Input: part model. Units: mm. Frame: model coordinates. Round coordinates to 2 decimals unless told otherwise and drop trailing zeros. Loops run counter-clockwise (first coordinate to the right, second up) from the corner with the lowest first, then second, coordinate; pieces in that order, holes last.
(1) Cut plane B-B, the plane x = 50.8. Output: boundary loops of the cut face in (y, z).
(2) Line query: line 1 (X direction, y = 22, z = 25.4); line 2 (X direction, y = 34.5, z = -27.5); line 3 (Z direction, x = -49, y = 22.5). Output: solid intervals per line, ascending.
(3) Cut plane A-A, the plane z = 25.4. Output: boundary loops of the cut face in (x, y), and give its area (3 significant figures).
(4) First-contact query: pin 1 Ø8.5 at (x, z) = (0, 0) entering from +Y. Flat tip, straight axial feed; report the tip coordinate or a pass-through.
from build123d import *

# Parameters (mm, degrees)
SKETCH1_W                                          = 152.4
SKETCH1_H                                          = 101.6
BOSS_EXTRUDE1_DEPTH                                = 76.2
CSK_FOR_10_FLAT_HEAD_MACHINE_SCREW_100_D           = 5.6134
CSK_FOR_10_FLAT_HEAD_MACHINE_SCREW_100_CSINK_D     = 9.779
CSK_FOR_10_FLAT_HEAD_MACHINE_SCREW_100_CSINK_ANGLE = 100
CSK_FOR_M6_FLAT_HEAD_MACHINE_SCREW1_D              = 6.4
CSK_FOR_M6_FLAT_HEAD_MACHINE_SCREW1_CSINK_D        = 12.6
CSK_FOR_M6_FLAT_HEAD_MACHINE_SCREW1_CSINK_ANGLE    = 90
F_7_16_14_TAPPED_HOLE3_D                           = 9.3472
F_7_16_14_TAPPED_HOLE3_DEPTH                       = 20.574
F_7_16_14_TAPPED_HOLE3_CSINK_D                     = 12.3825
F_7_16_14_TAPPED_HOLE3_CSINK_ANGLE                 = 90
F_7_16_14_TAPPED_HOLE3_TIP                         = 2.808182189
F_7_16_14_TAPPED_HOLE2_D                           = 9.3472


with BuildPart() as part:
    # Sketch1 → Boss-Extrude1 (new body)
    with BuildSketch(Plane(origin=(0, 0, 0), x_dir=(1, 0, 0), z_dir=(0, 1, 0))):
        Rectangle(SKETCH1_W, SKETCH1_H)
    extrude(amount=BOSS_EXTRUDE1_DEPTH)

    # CSK for #10 Flat Head Machine Screw (100)1 (through all)
    with Locations(Plane(origin=(0, 76.2, 0), x_dir=(1, 0, 0), z_dir=(0, 1, 0))):
        with Locations((-50.8, 25.4), (-50.8, -25.4), (50.8, -25.4), (50.8, 25.4)):
            CounterSinkHole(CSK_FOR_10_FLAT_HEAD_MACHINE_SCREW_100_D / 2, CSK_FOR_10_FLAT_HEAD_MACHINE_SCREW_100_CSINK_D / 2, counter_sink_angle=CSK_FOR_10_FLAT_HEAD_MACHINE_SCREW_100_CSINK_ANGLE)

    # CSK for M6 Flat Head Machine Screw1 (through all)
    with Locations(Plane(origin=(0, 76.2, 0), x_dir=(1, 0, 0), z_dir=(0, 1, 0))):
        with Locations((0, 0)):
            CounterSinkHole(CSK_FOR_M6_FLAT_HEAD_MACHINE_SCREW1_D / 2, CSK_FOR_M6_FLAT_HEAD_MACHINE_SCREW1_CSINK_D / 2, counter_sink_angle=CSK_FOR_M6_FLAT_HEAD_MACHINE_SCREW1_CSINK_ANGLE)

    # 7/16-14 Tapped Hole3
    with Locations(Plane(origin=(76.2, 0, 0), x_dir=(0, 0, -1), z_dir=(1, 0, 0))):
        with Locations((0, 38.1)):
            CounterSinkHole(F_7_16_14_TAPPED_HOLE3_D / 2, F_7_16_14_TAPPED_HOLE3_CSINK_D / 2, depth=F_7_16_14_TAPPED_HOLE3_DEPTH, counter_sink_angle=F_7_16_14_TAPPED_HOLE3_CSINK_ANGLE)
            with Locations((0, 0, -(F_7_16_14_TAPPED_HOLE3_DEPTH + F_7_16_14_TAPPED_HOLE3_TIP / 2))):  # 118° drill point
                Cone(0, F_7_16_14_TAPPED_HOLE3_D / 2, F_7_16_14_TAPPED_HOLE3_TIP, mode=Mode.SUBTRACT)

    # 7/16-14 Tapped Hole2 (through all)
    with Locations(Plane.XY.offset(50.8)):
        with Locations((0, 38.1)):
            Hole(F_7_16_14_TAPPED_HOLE2_D / 2)


solid = part.part
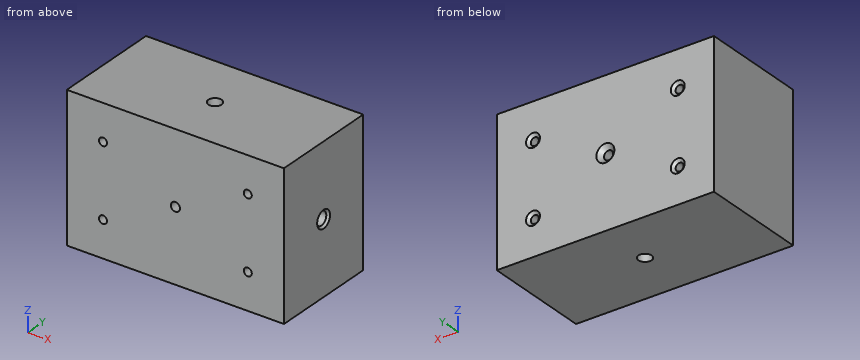
Reported:
1. outline: (0, -50.8) - (76.2, -50.8) - (76.2, -30.29) - (74.45, -28.21) - (0, -28.21) - close; (0, -22.59) - (74.45, -22.59) - (76.2, -20.51) - (76.2, 20.51) - (74.45, 22.59) - (0, 22.59) - close; (0, 28.21) - (74.45, 28.21) - (76.2, 30.29) - (76.2, 50.8) - (0, 50.8) - close
2. line 1: x = -76.2 to -53.61, -47.99 to 47.99, 53.61 to 76.2
2. line 2: x = -76.2 to -52.66, -48.94 to -2.98, 2.98 to 48.94, 52.66 to 76.2
2. line 3: z = -50.8 to -27.55, -23.25 to 23.25, 27.55 to 50.8
3. outline: (-76.2, 0) - (-53.61, 0) - (-53.61, 74.45) - (-55.69, 76.2) - (-76.2, 76.2) - close; (-47.99, 0) - (47.99, 0) - (47.99, 74.45) - (45.91, 76.2) - (-45.91, 76.2) - (-47.99, 74.45) - close; (53.61, 0) - (76.2, 0) - (76.2, 76.2) - (55.69, 76.2) - (53.61, 74.45) - close; hole circle Ø9.35 at (0, 38.1)
3. area: 10,700 mm2
4. pin 1: stops at y = 74.15
